Source: CAD feature listing. Evaluate the final solid. Frame: model axes, mm. Face numbers are marked on the shaded views. A direction names the side the tool comes from. Round coordinates to 2 decimals unless told otherwise and drop trailing zeros. Loops run counter-clockwise (first coordinate to the right, second up) from the corner with the lowest first, then second, coordinate; pieces in that order, holes last.
Item 1: Pull-direction query (Z, two-part tool) for the marked faces 4, 5 and 6; classes: released by +Z, released by -Z, zero draft, split by the parting line, or undercut.
Item 2: Access query for the marked faces 1, 2 and 3. Directions: +Z, -Z, +X, -X, +Y, -Y. A direction counts if a zero-diameter tool reaches every point of the face in a straight line with its end or side. Return the directions, or none.
Item 3: Ray query, L1, parallel to Y at x = -28, z = 0; L2, parallel to Y at x = -26.5, z = 0; L3, parallel to X at y = 92, z = 11.5. Return the intervals inside material, ascending.
Item 4: Section query B-B on z = 3.5. Return loops of the section in (x, y), then the cut area to 3 significant figures.
Item 5: First-contact query: P1, Ø4, axis at x = -75, z = 7.5, coming from the -Y side; P2, Ø2, axis at y = -25.5, z = -3.5, coming from the -X side; P3, Ø12.5, axis at y = -92.5, z = 4, coming from the -X side. Flat tips, straight axial feed; report the tip coordinate or a pass-through.
Item 6: Section query D-D on y = -65. Return loops of the section in (x, z).
Item 7: Section query A-A on y = -95. Return loops of the section in (x, z), then the cut area to 3 significant figures.
Item 8: Section query C-C on y = 0. Return loops of the section in (x, z).
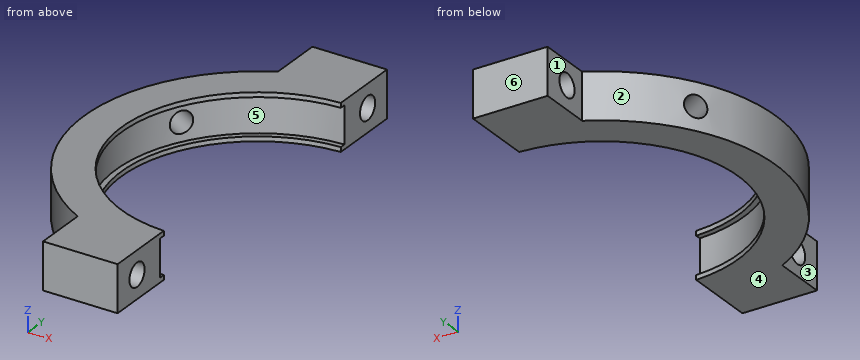
```python
from build123d import *

# Parameters (mm, degrees)
BOSS_EXTRUDE1_DEPTH    = 12.5
BOSS_EXTRUDE2_START    = 12.5
BOSS_EXTRUDE2_DEPTH    = 2.5
F_12_0MM_DOWEL_HOLE1_D = 12.5
G1_4_TAPPED_HOLE1_D    = 11.8


with BuildPart() as part:
    # Sketch1 → Boss-Extrude1 (new, symmetric)
    with BuildSketch(Plane.XY):
        with BuildLine():
            Line((-3, 75.940766391), (-3, 92.951600309))
            ThreePointArc((-3, 92.951600309), (-23.590407766, 89.958282895), (-43, 82.462112512))
            ThreePointArc((-43, 82.462112512), (-93, 0), (-43, -82.462112512))
            ThreePointArc((-43, -82.462112512), (-23.590407766, -89.958282895), (-3, -92.951600309))
            Line((-3, -92.951600309), (-3, -75.940766391))
            ThreePointArc((-3, -75.940766391), (-76, 0), (-3, 75.940766391))
        make_face()
        with BuildLine():
            Line((-3, 92.951600309), (-3, 111))
            Line((-3, 111), (-43, 111))
            Line((-43, 111), (-43, 82.462112512))
            ThreePointArc((-43, 82.462112512), (-23.590407766, 89.958282895), (-3, 92.951600309))
        make_face()
        with BuildLine():
            ThreePointArc((-3, -92.951600309), (-23.590407766, -89.958282895), (-43, -82.462112512))
            Line((-43, -82.462112512), (-43, -111))
            Line((-43, -111), (-3, -111))
            Line((-3, -111), (-3, -92.951600309))
        make_face()
    extrude(amount=BOSS_EXTRUDE1_DEPTH, both=True)

    # Sketch1_3 → Boss-Extrude2 (add)
    with BuildSketch(Plane.XY.offset(BOSS_EXTRUDE2_START)):
        with BuildLine():
            Line((-3, 72.938330115), (-3, 75.940766391))
            ThreePointArc((-3, 75.940766391), (-76, 0), (-3, -75.940766391))
            Line((-3, -75.940766391), (-3, -72.938330115))
            ThreePointArc((-3, -72.938330115), (-73, 0), (-3, 72.938330115))
        make_face()
    boss_extrude2 = extrude(amount=-BOSS_EXTRUDE2_DEPTH)

    # 12.0mm Dowel Hole1 (through all)
    with Locations(Plane(origin=(-3, 0, 0), x_dir=(0, 0, -1), z_dir=(1, 0, 0))):
        with Locations((0, 95), (0, -95)):
            Hole(F_12_0MM_DOWEL_HOLE1_D / 2)

    # Mirror2: Boss-Extrude2 across plane
    add(boss_extrude2.mirror(Plane.XY))

    # G1_4 Tapped Hole1 (through all)
    with Locations(Plane(origin=(-80.540362552, 46.5, 0), x_dir=(0, 0, 1), z_dir=(-0.8660254037844382, 0.500000000000001, 0))):
        with Locations((0, 0)):
            Hole(G1_4_TAPPED_HOLE1_D / 2)


solid = part.part
```
Data:
1. face 4: released by -Z
1. face 5: undercut
1. face 6: zero draft
2. face 1: +Z, -Z, -X, +Y
2. face 2: +Z, -Z, -X
2. face 3: +Z, -Z, -X, -Y
3. L1: y = -111 to -101.25, -88.75 to -70.65, 70.65 to 88.75, 101.25 to 111
3. L2: y = -111 to -101.25, -88.75 to -71.23, 71.23 to 88.75, 101.25 to 111
3. L3: x = -43 to -3
4. outline: (-82.81, 42.33) arc R93 ccw to (-43, -82.46) - (-43, -89.82) - (-3, -89.82) - (-3, -75.94) arc R76 cw to (-68.06, 33.81) - close; (-78.06, 50.55) - (-63.31, 42.04) arc R76 cw to (-3, 75.94) - (-3, 89.82) - (-43, 89.82) - (-43, 82.46) arc R93 ccw to start; (-43, -111) - (-3, -111) - (-3, -100.18) - (-43, -100.18) - close; (-43, 100.18) - (-3, 100.18) - (-3, 111) - (-43, 111) - close
4. area: 5,160 mm2
5. P1: stops at y = -57.62
5. P2: stops at x = -89.71
5. P3: stops at x = -43
6. outline: (-66.51, -12.5) - (-33.23, -12.5) - (-33.23, -10) - (-39.38, -10) - (-39.38, 10) - (-33.23, 10) - (-33.23, 12.5) - (-66.51, 12.5) - close
7. outline: (-43, -12.5) - (-3, -12.5) - (-3, -6.25) - (-43, -6.25) - close; (-43, 6.25) - (-3, 6.25) - (-3, 12.5) - (-43, 12.5) - close
7. area: 500 mm2
8. outline: (-93, -12.5) - (-73, -12.5) - (-73, -10) - (-76, -10) - (-76, 10) - (-73, 10) - (-73, 12.5) - (-93, 12.5) - close
